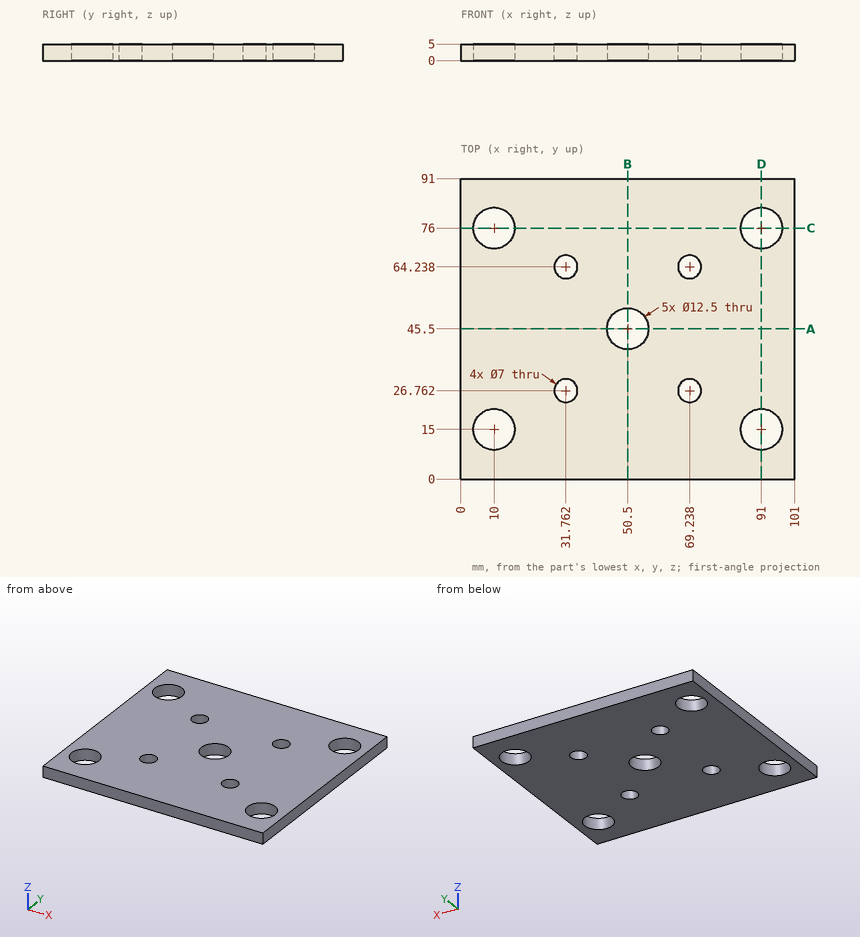
Verification items for this drawing (mm, ordinates from the low corner). Give positions to 0.01 mm unless a question says otherwise; leave off trailing zeros. Loops run counter-clockwise (first coordinate to the right, second up) from the corner with the lowest first, then second, coordinate; pieces in that order, holes last.
1. Cross-section at C-C on y = 76. Record the cut outline in (x, z).
Derived:
outline: (0, 0) - (3.75, 0) - (3.75, 5) - (0, 5) - close; (16.25, 0) - (84.75, 0) - (84.75, 5) - (16.25, 5) - close; (97.25, 0) - (101, 0) - (101, 5) - (97.25, 5) - close
2. Material ranges on probe 1 along Y at (x, z) = (10, 3.05); probe 2 along X at (y, z) = (62.5, 0.35) (1 decimal); probe 3 along Y at (x, z) = (86, 1.1), recorded low to high.
Derived:
probe 1: y = 0 to 8.75, 21.25 to 69.75, 82.25 to 91
probe 2: x = 0 to 28.7, 34.8 to 66.2, 72.3 to 101
probe 3: y = 0 to 11.25, 18.75 to 72.25, 79.75 to 91
3. Cross-section at B-B on x = 50.5. Record the cut outline in (y, z).
Derived:
outline: (0, 0) - (39.25, 0) - (39.25, 5) - (0, 5) - close; (51.75, 0) - (91, 0) - (91, 5) - (51.75, 5) - close
4. Cross-section at A-A on y = 45.5. Record the cut outline in (x, z).
Derived:
outline: (0, 0) - (44.25, 0) - (44.25, 5) - (0, 5) - close; (56.75, 0) - (101, 0) - (101, 5) - (56.75, 5) - close
5. Cross-section at D-D on x = 91. Record the cut outline in (y, z).
Derived:
outline: (0, 0) - (8.75, 0) - (8.75, 5) - (0, 5) - close; (21.25, 0) - (69.75, 0) - (69.75, 5) - (21.25, 5) - close; (82.25, 0) - (91, 0) - (91, 5) - (82.25, 5) - close
